Could you check a few things on this model? Use its own coordinates, in mm. Face numbers are marked on the shaded views. A direction names the side the tool comes from. Coordinates: 2 decimals unless noted, no trailing zeros. Write each loop counter-clockwise with the first axis right and the second up, starting at its lowest first coordinate (ties: lowest second). Pieces come first, ordered by that corner, then holes. Notation, with made-up numbers: M -15,27.25 L 31,27.25 A11 ccw 31,44.25 Z; hole C -6.5,-19.75 d11. An arc over 180 degrees is marked long. Answer as CSV lines item,"result". Start each with the question number.
Item 1: On a 3-axis mill with a long thin cutter (end or side, diameter ignored), from which of +Z, -Z, +X, -X, +Y, -Y can I reach the whole of each face in a straight line? I mean the marked faces 1 and 2. Say none if no direction works.
Item 2: Suppose I cut it at B-B, the plane x = -59.5. Write out the boundary of the cut face in (y, z), and give its area (3 significant figures).
Item 3: Suppose I cut it at A-A, the plane z = 45.5. Write out the boundary of the cut face in (x, y).
Item 4: We'd pull the mould along Z, two halves only. Please class the marked faces 3, 4, 5 and 6: +Z half, -Z half, draft (parallel to the pull), parting line (faces both ways), or undercut.
Item 5: Suppose I cut it at D-D, the plane y = -5.5. Write out the boundary of the cut face in (x, z).
Item 6: Suppose I cut it at C-C, the plane y = -30.5. Write out the boundary of the cut face in (x, z), and give its area (3 significant figures).
Item 7: I'm going to push a flat-ended pin straight in: P1, Ø1.6, axis at x = -57, y = -35, coming from the +Z side. Where does the tip first touch, or does it pass through?
Item 8: If I drill on line 1 along Z through (x, y) = (-44.5, -19.5); line 2 along Z through (x, y) = (-60.5, -33.5); line 3 along X through (y, z) = (-2.5, 50.5), over which ranges is the centre line in solid material (lowest first)? Write a range as [from, to].
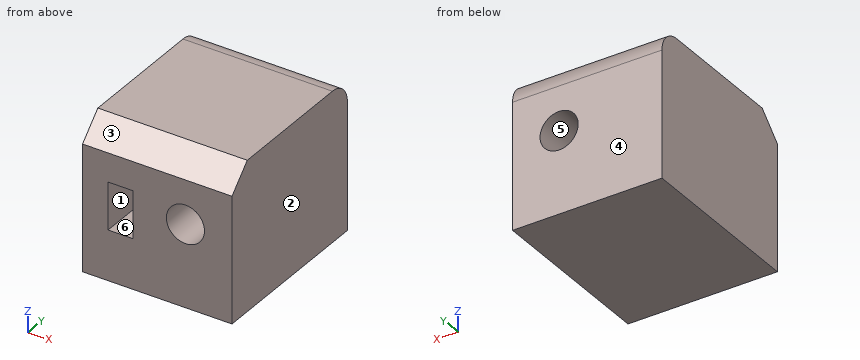
```python
from build123d import *

# Parameters (mm, degrees)
F0_W     = 32.591233
F0_H     = 32.591233
F1_DEPTH = 38.354
F2_SIZE  = 5.08
F3_R     = 4.158382
F4_DEPTH = 40.132
F5_W     = 5.479913
F5_H     = 10.327767
F6_DEPTH = 9.906
F7_R     = 5


with BuildPart() as f1:
    # F0 (on Front) → F1 (new body)
    with BuildSketch(Plane.XZ):
        with Locations((-50.354915, 45.510276)):
            Rectangle(F0_W, F0_H)
    extrude(amount=F1_DEPTH)

    # F2
    f2_edges = [f1.edges().sort_by_distance(p)[0] for p in [
        (-50.354916, -38.354, 61.805893),
    ]]
    chamfer(f2_edges, length=F2_SIZE)

    # F3 (on face) → F4 (cut)
    with BuildSketch(Plane.XZ):
        with Locations((-44.212125, 47.174979)):
            Circle(F3_R)
    extrude(amount=F4_DEPTH, mode=Mode.SUBTRACT)

    # F5 (on face) → F6 (cut)
    with BuildSketch(Plane.XZ.offset(38.354)):
        with Locations((-58.341155, 45.296827)):
            Rectangle(F5_W, F5_H)
    extrude(amount=-F6_DEPTH, mode=Mode.SUBTRACT)

    # F7
    f7_edges = [f1.edges().sort_by_distance(p)[0] for p in [
        (-50.354916, 0, 61.805893),
    ]]
    fillet(f7_edges, radius=F7_R)


solid = f1.part
```
Ans:
1,face 1,"-Y"
1,face 2,"+Z, -Z, +X, +Y, -Y"
2,outline,"M -38.35,29.21 L 0,29.21 L 0,56.81 A5 ccw -5,61.81 L -33.27,61.81 L -38.35,56.73 L -38.35,50.46 L -28.45,50.46 L -28.45,40.13 L -38.35,40.13 Z"
2,area,"1,130 mm^2"
3,outline,"M -66.65,-38.35 L -61.08,-38.35 L -61.08,-28.45 L -55.6,-28.45 L -55.6,-38.35 L -48.02,-38.35 L -48.02,0 L -66.65,0 Z; M -40.41,-38.35 L -34.06,-38.35 L -34.06,0 L -40.41,0 Z"
4,face 3,"+Z half"
4,face 4,"draft"
4,face 5,"undercut"
4,face 6,"undercut"
5,outline,"M -66.65,29.21 L -34.06,29.21 L -34.06,61.81 L -66.65,61.81 Z; hole C -44.21,47.17 d8.32"
6,outline,"M -66.65,29.21 L -34.06,29.21 L -34.06,61.81 L -66.65,61.81 Z; hole M -61.08,40.13 L -55.6,40.13 L -55.6,50.46 L -61.08,50.46 Z; hole C -44.21,47.17 d8.32"
6,area,"951 mm^2"
7,P1,"stops at z = 60.88"
8,line 1,"z = [29.21, 43.03], [51.32, 61.81]"
8,line 2,"z = [29.21, 40.13], [50.46, 61.58]"
8,line 3,"x = [-66.65, -46.71], [-41.71, -34.06]"
